from build123d import *

# Parameters (mm, degrees)
BOSS_EXTRUDE1_DEPTH = 10
FILLET1_R           = 5
SKETCH2_R           = 3
CUT_EXTRUDE1_DEPTH  = 15


with BuildPart() as part:
    # Sketch1 → Boss-Extrude1 (new body)
    with BuildSketch(Plane.XY):
        Polygon((-169.15, 40.054759159), (169.15, 40.054759159), (215.74113672, -41.201675672), (-169.15, -40.054759159), align=None)
    extrude(amount=BOSS_EXTRUDE1_DEPTH)

    # Fillet1
    fillet1_edges = [part.edges().sort_by_distance(p)[0] for p in [
        (-169.15, 40.054759159, 5),
        (169.15, 40.054759159, 5),
        (215.74113672, -41.201675672, 5),
        (-169.15, -40.054759159, 5),
    ]]
    fillet(fillet1_edges, radius=FILLET1_R)

    # Sketch2 → Cut-Extrude1 (cut)
    with BuildSketch(Plane(origin=(0, 0, 0), x_dir=(-1, 0, 0), z_dir=(0, 0, -1))):
        with Locations((144.15, 30.054759159)):
            Circle(SKETCH2_R)
        with Locations((159.15, 30.054759159)):
            Circle(SKETCH2_R)
        with Locations((159.15, 18.054759159)):
            Circle(SKETCH2_R)
        with Locations((159.15, 6.054759159)):
            Circle(SKETCH2_R)
        with Locations((144.15, 18.054759159)):
            Circle(SKETCH2_R)
        with Locations((144.15, 6.054759159)):
            Circle(SKETCH2_R)
        with Locations((144.149466916, -6.067437377)):
            Circle(SKETCH2_R)
        with Locations((144.148411495, -18.06743733)):
            Circle(SKETCH2_R)
        with Locations((159.149466858, -6.068756652)):
            Circle(SKETCH2_R)
        with Locations((159.148411437, -18.068756606)):
            Circle(SKETCH2_R)
        with Locations((159.147356017, -30.06875656)):
            Circle(SKETCH2_R)
        with Locations((144.147356075, -30.067437284)):
            Circle(SKETCH2_R)
        with Locations((-165.763069515, 26.671271591)):
            Circle(SKETCH2_R)
        with Locations((-195.608099644, -25.379416941)):
            Circle(SKETCH2_R)
        with Locations((-190.633927956, -16.704302185)):
            Circle(SKETCH2_R)
        with Locations((-185.659756267, -8.02918743)):
            Circle(SKETCH2_R)
        with Locations((-180.685584579, 0.645927325)):
            Circle(SKETCH2_R)
        with Locations((-175.711412891, 9.32104208)):
            Circle(SKETCH2_R)
        with Locations((-170.737241203, 17.996156836)):
            Circle(SKETCH2_R)
        with Locations((-200.582271332, -34.054531696)):
            Circle(SKETCH2_R)
    extrude(amount=-CUT_EXTRUDE1_DEPTH, mode=Mode.SUBTRACT)


solid = part.part
Geometry check sheet. Reference: the model listing, model coordinates, mm. Round coordinates to 2 decimals unless told otherwise and drop trailing zeros.
Item 1: Gauge pin test, flat ends, axial feed: pin 1 (1.5 mm diameter, centred on y = -2, z = 1, fed in from +X); pin 2 (5.5 mm diameter, centred on x = 170.74, y = 18, fed in from -Z); pin 3 (3 mm diameter, centred on y = 32, z = 1.5, fed in from +X). Record the tip position at first contact, or that the pin passes through.
Item 2: Thickness scan on line 1 (X direction, y = -18, z = 5.25); line 2 (X direction, y = 30, z = 7.5); line 3 (X direction, y = -1, z = 2.25). Record the ranges inside material, lowest first.
Item 3: Mould release check, pull along Y, two halves, no side actions. Record for faces 1 (the flat face through (-1, 40.055, 5)), 2 (the cylindrical face through (-147.01, -29.17, 4.93)), 3 (the flat face through (-169.15, 0, 5)), 4 (the cylindrical face through (-160.763, 32.584, 4.93)): pulls with the +Y half, pulls with the -Y half, needs draft (parallel to the pull), parting line crosses it, or undercut.
Item 4: Cross-section at A-A on z = 7.5. Count the separate pieces of the cut face and the enclosed holes in it, then the cut area to 3 significant figures.
Answer sheet:
1. pin 1: stops at x = 193.69
1. pin 2: passes through
1. pin 3: stops at x = 174.63
2. line 1: x = -169.15 to -162.15, -156.15 to -147.15, -141.15 to 187.93, 193.34 to 202.44
2. line 2: x = -169.15 to -162.15, -156.15 to -147.15, -141.15 to 174.92
2. line 3: x = -169.15 to 178.18, 183.19 to 192.69
3. face 1: pulls with the +Y half
3. face 2: undercut
3. face 3: needs draft
3. face 4: undercut
4. separate pieces: 1
4. enclosed holes: 20
4. area: 28,600 mm2
